Verification items for the finished model (mm, model axes). A direction names the side the tool comes from. Coordinates: 2 decimals unless noted, no trailing zeros. Loops run counter-clockwise (first coordinate to the right, second up) from the corner with the lowest first, then second, coordinate; pieces in that order, holes last. Notation, with made-up numbers: (-28.75, 74) -> (10.25, 74) arc R25 cw to (10.25, 112) -> close; hole circle Ø5 at (87, -3.75). An arc over 180 degrees is marked (long way). Answer as a JSON object with one key per item and string values. Group by question number.
Q1. Release check for a two-part mould opening along X. For faces 4 (the flat face through (2.25, 0, -2)), 5 (the flat face through (3, 0, -4.5)), 6 (the flat face through (-3.45, 0, -2)) record: released by +X, released by -X, zero draft, split by the parting line, or undercut.
Q2. Cross-section at B-B on x = 8. Record the boundary of the cut face in (y, z), and give its area (3 significant figures).
Q3. Gauge pin test, flat ends, axial feed: pin 1 Ø3 at (y, z) = (-0.5, -2) entering from +X; pin 2 Ø1.5 at (x, z) = (1.5, -0.5) entering from +Y; pin 3 Ø0.8 at (y, z) = (-0.5, -2.5) entering from -X; pin 4 Ø0.6 at (x, z) = (-3, -3) entering from -Y. Record the tip position at first contact, or that the pin passes through.
Q4. Set-up check for faces 1 (the flat face through (-2.25, 0, -2)), 2 (the flat face through (-3, 0, -4.5)), 3 (the flat face through (3.45, 0, -2)): record each of +Z, -Z, +X, -X, +Y, -Y from which the full face is reachable in a straight line by a thin tool's end or side.
Q5. Cross-section at D-D on y = -7.5. Record the boundary of the cut face in (x, z) (3 decimals), and give its area (3 significant figures).
Q6. Cross-section at A-A on z = -3.5. Record the boundary of the cut face in (x, y), and give its area (3 significant figures).
Q7. Cross-section at C-C on y = 0.5. Record the boundary of the cut face in (x, z) (3 decimals), and give its area (3 significant figures).
Q8. Scan lines: L1, parallel to X at y = -1.25, z = -2.75; L2, parallel to Z at x = -5.5, y = 3.75. Record each from-to range of solid material in increasing order.
```python
from build123d import *

# Parameters (mm, degrees)
SKETCH_W        = 37.05
SKETCH_H        = 18
PAD_DEPTH       = 2
CHAMFER_SIZE    = 1
FILLET_R        = 1
SKETCH001_W     = 1.2
SKETCH001_H     = 3
PAD001_DEPTH    = 4.5
CHAMFER001_SIZE = 0.2


with BuildPart() as part:
    # Sketch → Pad (new body)
    with BuildSketch(Plane.XY):
        Rectangle(SKETCH_W, SKETCH_H)
    extrude(amount=PAD_DEPTH)

    # Chamfer
    chamfer_edges = [part.edges().sort_by_distance(p)[0] for p in [
        (-18.525, 0, 2),
        (0, 9, 2),
        (18.525, 0, 2),
        (0, -9, 2),
    ]]
    chamfer(chamfer_edges, length=CHAMFER_SIZE)

    # Fillet
    fillet_edges = [part.edges().sort_by_distance(p)[0] for p in [
        (0, -9, 1),
        (18.525, 0, 1),
        (-18.525, 0, 1),
        (0, 9, 1),
    ]]
    fillet(fillet_edges, radius=FILLET_R)

    # Sketch001 (on Face4 of Fillet) → Pad001 (join)
    with BuildSketch(Plane(origin=(0, 0, 0), x_dir=(1, 0, 0), z_dir=(0, 0, -1))):
        with Locations((-2.85, 0)):
            Rectangle(SKETCH001_W, SKETCH001_H)
        with Locations((2.85, 0)):
            Rectangle(SKETCH001_W, SKETCH001_H)
    extrude(amount=PAD001_DEPTH)

    # Chamfer001
    chamfer001_edges = [part.edges().sort_by_distance(p)[0] for p in [
        (2.85, 1.5, -4.5),
        (3.45, 0, -4.5),
        (2.85, -1.5, -4.5),
        (2.25, 0, -4.5),
        (3.45, 1.5, -2.25),
        (2.25, 1.5, -2.25),
        (3.45, -1.5, -2.25),
        (2.25, -1.5, -2.25),
        (-2.25, 0, -4.5),
        (-2.85, -1.5, -4.5),
        (-3.45, 0, -4.5),
        (-2.85, 1.5, -4.5),
        (-2.25, -1.5, -2.25),
        (-3.45, -1.5, -2.25),
        (-3.45, 1.5, -2.25),
        (-2.25, 1.5, -2.25),
    ]]
    chamfer(chamfer001_edges, length=CHAMFER001_SIZE)


solid = part.part
```
Computed values:
{
 "1": {"face 4": "undercut", "face 5": "zero draft", "face 6": "released by -X"},
 "2": {"outline": "(-9, 0) -> (9, 0) -> (9, 0.59) arc R1 ccw to (8.71, 1.29) -> (8, 2) -> (-8, 2) -> (-8.71, 1.29) arc R1 ccw to (-9, 0.59) -> close", "area": "35.0 mm²"},
 "3": {"pin 1": "stops at x = 3.45", "pin 2": "stops at y = 9", "pin 3": "stops at x = -3.45", "pin 4": "stops at y = -1.5"},
 "4": {"face 1": "-Z, +Y, -Y", "face 2": "-Z, +X, -X, +Y, -Y", "face 3": "-Z, +X, +Y, -Y"},
 "5": {"outline": "(-18.525, 0) -> (18.525, 0) -> (18.525, 0.586) arc R1 ccw to (18.232, 1.293) -> (17.525, 2) -> (-17.525, 2) -> (-18.232, 1.293) arc R1 ccw to (-18.525, 0.586) -> close", "area": "73.1 mm²"},
 "6": {"outline": "(-3.45, -1.3) -> (-3.25, -1.5) -> (-2.45, -1.5) -> (-2.25, -1.3) -> (-2.25, 1.3) -> (-2.45, 1.5) -> (-3.25, 1.5) -> (-3.45, 1.3) -> close; (2.25, -1.3) -> (2.45, -1.5) -> (3.25, -1.5) -> (3.45, -1.3) -> (3.45, 1.3) -> (3.25, 1.5) -> (2.45, 1.5) -> (2.25, 1.3) -> close", "area": "7.04 mm²"},
 "7": {"outline": "(-18.525, 0) -> (-3.45, 0) -> (-3.45, -4.3) -> (-3.25, -4.5) -> (-2.45, -4.5) -> (-2.25, -4.3) -> (-2.25, 0) -> (2.25, 0) -> (2.25, -4.3) -> (2.45, -4.5) -> (3.25, -4.5) -> (3.45, -4.3) -> (3.45, 0) -> (18.525, 0) -> (18.525, 0.586) arc R1 ccw to (18.232, 1.293) -> (17.525, 2) -> (-17.525, 2) -> (-18.232, 1.293) arc R1 ccw to (-18.525, 0.586) -> close", "area": "83.8 mm²"},
 "8": {"L1": "x = -3.45 to -2.25, 2.25 to 3.45", "L2": "z = 0 to 2"}
}
